The model under review builds one solid part; all positions refer to its coordinate system, in mm. A direction names the side the tool comes from. Coordinates: 2 decimals unless noted, no trailing zeros. Order: outer loops, then holes, each group sorted by start corner. A loop starts at its lowest first (then second) coordinate and runs counter-clockwise, first axis right, second up. Notation, with made-up numbers: M -30,-9 L 24,-9 A28 cw 24,25 Z; hole C 21.25,-15 d5. An arc over 180 degrees is marked long. Write each question's results on one line, items separated by ' | '.
from build123d import *

# Parameters (mm, degrees)
BOSS_EXTRU_1_DEPTH = 5
CONG_1_R           = 2


with BuildPart() as part:
    # Esquisse1 → Boss.-Extru.1 (new body)
    with BuildSketch(Plane.XY):
        Polygon((0, 0), (71, 0), (76, 0), (76, 5), (71, 5), (71, 16.5), (76, 16.5), (76, 21.5), (71, 21.5), (71, 33), (76, 33), (76, 38), (71, 38), (0, 38), (-5, 38), (-5, 33), (0, 33), (0, 5), (-5, 5), (-5, 0), align=None)
        Polygon((39, 28), (59, 28), (59, 10), (39, 10), (39, 19), (29, 19), (29, 28), align=None, mode=Mode.SUBTRACT)
    extrude(amount=BOSS_EXTRU_1_DEPTH)

    # Congé1
    cong_1_edges = [part.edges().sort_by_distance(p)[0] for p in [
        (29, 28, 2.5),
        (29, 19, 2.5),
        (39, 19, 2.5),
        (39, 10, 2.5),
        (59, 10, 2.5),
        (59, 28, 2.5),
    ]]
    fillet(cong_1_edges, radius=CONG_1_R)


solid = part.part
1) Take a section at C-C on z = 2.2. State the section outline as (x, y) points, plus the area to 3 significant figures.
Solutions:
outline: M -5,0 L 76,0 L 76,5 L 71,5 L 71,16.5 L 76,16.5 L 76,21.5 L 71,21.5 L 71,33 L 76,33 L 76,38 L -5,38 L -5,33 L 0,33 L 0,5 L -5,5 Z; hole M 29,21 A2 ccw 31,19 L 37,19 A2 cw 39,17 L 39,12 A2 ccw 41,10 L 57,10 A2 ccw 59,12 L 59,26 A2 ccw 57,28 L 31,28 A2 ccw 29,26 Z | area: 2,380 mm2
2) For pin 1 (1 mm diameter, centred on x = 10, z = 2.5, fed in from -Y); pin 2 (3 mm diameter, centred on y = 30.5, z = 1, fed in from +X), all flat-tipped, find the tip position at first contact; note any pin that passes through.
Solutions:
pin 1: y = 0 | pin 2: x = 71
3) For faces 5 (the flat face through (76, 19, 2)), 6 (the flat face through (35, 15, 5)), 7 (the flat face through (0, 19, 2)), 8 (the flat face through (59, 19, 2)), 9 (the flat face through (71, 11, 2)), list the 3-axis set-ups (+Z, -Z, +X, -X, +Y, -Y) from which the entire face can be reached by the end or side of a thin tool; tool diameter is ignored.
Solutions:
face 5: +Z, -Z, +X, +Y, -Y | face 6: +Z, +X, -X, +Y, -Y | face 7: +Z, -Z, -X | face 8: +Z, -Z | face 9: +Z, -Z, +X
4) Take a section at B-B on y = 13.5. State the section outline as (x, z) points.
Solutions:
outline: M 0,0 L 39,0 L 39,5 L 0,5 Z; M 59,0 L 71,0 L 71,5 L 59,5 Z
5) The part is to be moulded in two halves that separate along Y. For faces 1 (the flat face through (-2, 5, 2)), 2 (the flat face through (36, 38, 2)), 3 (the flat face through (76, 2, 2)), 4 (the cylindrical face through (29.6, 19.57, 2.54)), say which applies: pulls with the +Y half, pulls with the -Y half, needs draft (parallel to the pull), parting line crosses it, or undercut.
Solutions:
face 1: undercut | face 2: pulls with the +Y half | face 3: needs draft | face 4: undercut
6) Take a section at A-A on x = 32.5. State the section outline as (y, z) points, plus the area to 3 significant figures.
Solutions:
outline: M 0,0 L 19,0 L 19,5 L 0,5 Z; M 28,0 L 38,0 L 38,5 L 28,5 Z | area: 145 mm2
7) Take a section at D-D on y = 8.5. State the section outline as (x, z) points, plus the area to 3 significant figures.
Solutions:
outline: M 0,0 L 71,0 L 71,5 L 0,5 Z | area: 355 mm2
8) To check wall thickness, follow line 1 along X through (y, z) = (14, 4.75); line 2 along X through (y, z) = (23.5, 1.55); line 3 along Y through (x, z) = (55.5, 4.25). State the ranges of each line that lie inside material, in increasing order.
Solutions:
line 1: 0 to 39, 59 to 71 | line 2: 0 to 29, 59 to 71 | line 3: 0 to 10, 28 to 38
